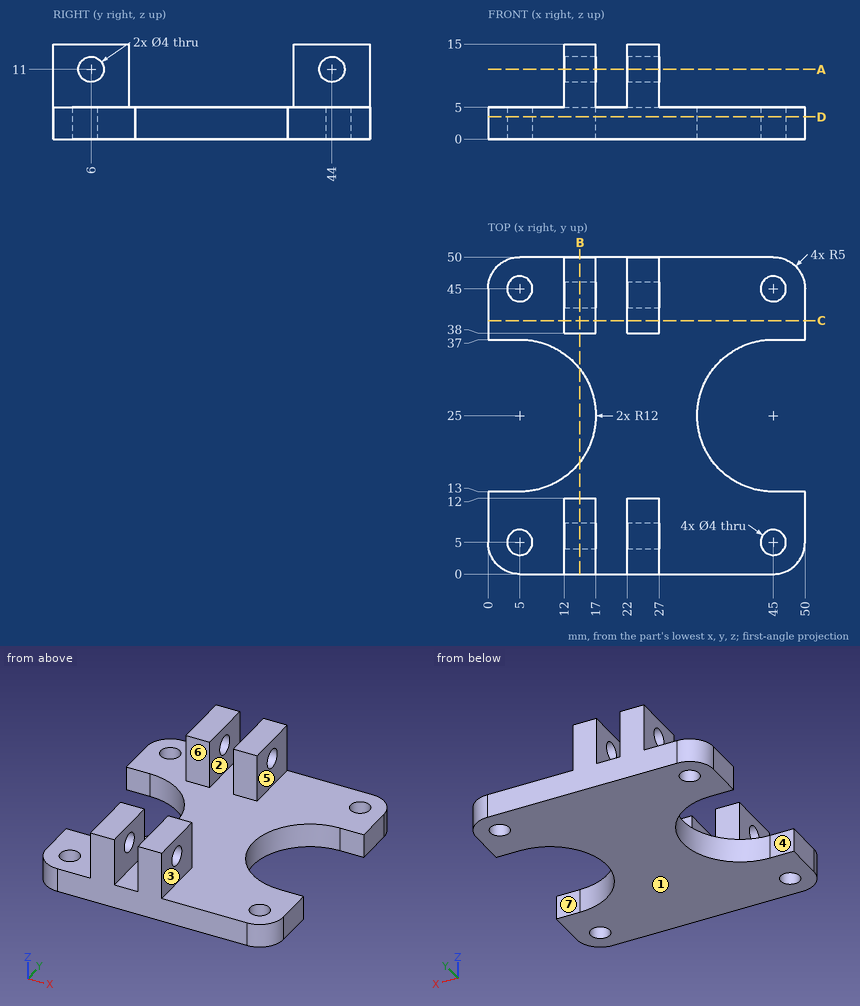
Here's the drawing with two shaded views (mm, measured from the low corner). I have some questions. A direction names the side the tool comes from. Coordinates: 2 decimals unless noted, no trailing zeros. Write each loop counter-clockwise with the first axis right and the second up, starting at its lowest first coordinate (ties: lowest second). Pieces come first, ordered by that corner, then holes. Notation, with made-up numbers: (88.5, -3) -> (140.5, -3) arc R28 cw to (140.5, 33) -> close; hole circle Ø1 at (57, 24). An arc over 180 degrees is marked (long way). Use a Markdown table: item, result. Add a question column.
(1) If we section it at A-A, the plane z = 11: State how many separate pieces and enclosed holes the cut face has, and give its area (3 significant figures).
(2) If we section it at B-B, the plane x = 14.5: Write out the boundary of the cut face in (y, z), and give its area (3 significant figures).
(3) Please list where these lines run through material, in increasing order: line 1 (Y direction, x = 5, z = 1.15); line 2 (Z direction, x = 15.8, y = 44); line 3 (Y direction, x = 45.5, z = 1).
(4) We'd pull the mould along X, two halves only. Please class the marked faces 1, 2 and 3: +X half, -X half, draft (parallel to the pull), parting line (faces both ways), or undercut.
(5) I'm going to push flat-ended pins straight in: P1, Ø8, axis at y = 27, z = 3.5, coming from the +X side; P2, Ø5, axis at y = 44, z = 11, coming from the +X side; P3, Ø5, axis at y = 3, z = 11.5, coming from the -X side. Where does each tip first touch, or does it pass through?
(6) For the marked faces 4, 5, 6 and 7, which set-ups out of +Z, -Z, +X, -X, +Y, -Y let a thin tool reach every point of the face, with its end or its side?
(7) If we section it at D-D, the plane z = 3.5: Write out the boundary of the cut face in (x, y), and give its area (3 significant figures).
(8) If we section it at C-C, the plane y = 40: Write out the boundary of the cut face in (x, z), and give its area (3 significant figures).
Outcome:
| question | item | result |
|---|---|---|
| 1 | separate pieces | 8 |
| 1 | enclosed holes | 0 |
| 1 | area | 160 mm^2 |
| 2 | outline | (0, 0) -> (17.67, 0) -> (17.67, 5) -> (12, 5) -> (12, 15) -> (0, 15) -> close; (32.33, 0) -> (50, 0) -> (50, 15) -> (38, 15) -> (38, 5) -> (32.33, 5) -> close; hole circle Ø4 at (6, 11); hole circle Ø4 at (44, 11) |
| 2 | area | 392 mm^2 |
| 3 | line 1 | y = 0 to 3, 7 to 13, 37 to 43, 47 to 50 |
| 3 | line 2 | z = 0 to 9, 13 to 15 |
| 3 | line 3 | y = 0.03 to 3.06, 6.94 to 13, 37 to 43.06, 46.94 to 49.97 |
| 4 | face 1 | draft |
| 4 | face 2 | undercut |
| 4 | face 3 | +X half |
| 5 | P1 | stops at x = 34.61 |
| 5 | P2 | stops at x = 27 |
| 5 | P3 | stops at x = 12 |
| 6 | face 4 | +Z, -Z, -X |
| 6 | face 5 | +Z, +X, +Y, -Y |
| 6 | face 6 | +Z, +X, -X |
| 6 | face 7 | +Z, -Z, +X |
| 7 | outline | (0, 5) arc R5 ccw to (5, 0) -> (45, 0) arc R5 ccw to (50, 5) -> (50, 13) -> (45, 13) arc R12 cw to (45, 37) -> (50, 37) -> (50, 45) arc R5 ccw to (45, 50) -> (5, 50) arc R5 ccw to (0, 45) -> (0, 37) -> (5, 37) arc R12 cw to (5, 13) -> (0, 13) -> close; hole circle Ø4 at (5, 5); hole circle Ø4 at (5, 45); hole circle Ø4 at (45, 5); hole circle Ø4 at (45, 45) |
| 7 | area | 1,740 mm^2 |
| 8 | outline | (0, 0) -> (50, 0) -> (50, 5) -> (27, 5) -> (27, 15) -> (22, 15) -> (22, 5) -> (17, 5) -> (17, 15) -> (12, 15) -> (12, 5) -> (0, 5) -> close |
| 8 | area | 350 mm^2 |
